```python
from build123d import *

# Parameters (mm, degrees)
F0_R        = 3
F1_DEPTH    = 3
F2_R        = 10
F3_R        = 5
F4_R        = 1
F5_T1_DEPTH = 3
F6_R        = 20
F7_R        = 1
F8_R        = 3
F9_R        = 8


# Not quite as in the source:
# - a fillet or chamfer that OpenCascade refuses, or shapes differently, is made with other operations: its cross-section is extruded or revolved along the edge and cut away or added
# - a feature names something its author has since deleted; it is built from what else it names


with BuildPart() as f1:
    # F0 (on Front) → F1 (new body)
    with BuildSketch(Plane.XZ):
        Polygon((-2, -2), (1.3333333333, 0), (0, 0), (0, 7), (-10, 2.5), (-10, -2), align=None)
        Polygon((14.2307692308, 0), (32, 0), (40, 0), (40, 7), (0, 7), (0, 0), (1.3333333333, 0), (8, 4), (13, 4), align=None)
        Polygon((15, -5), (32, 0), (14.2307692308, 0), (15, -2.5), (11.75, -3.5), align=None)
        with BuildLine():
            Line((40, 7), (40, 0))
            ThreePointArc((40, 0), (61.4283268073, 3.5), (40, 7))
        make_face()
        with Locations((57.4283268073, 3.5)):
            Circle(F0_R, mode=Mode.SUBTRACT)
    extrude(amount=F1_DEPTH)

    # F2
    f2_edges = [f1.edges().sort_by_distance(p)[0] for p in [
        (32, -1.5, 0),
    ]]
    fillet(f2_edges, radius=F2_R)

    # F3
    f3_edges = [f1.edges().sort_by_distance(p)[0] for p in [
        (13, -1.5, 4),
        (-2, -1.5, -2),
    ]]
    fillet(f3_edges, radius=F3_R)

    # F4
    f4_edges = [f1.edges().sort_by_distance(p)[0] for p in [
        (15, -1.5, -2.5),
    ]]
    fillet(f4_edges, radius=F4_R)

    # F5: fillet of radius 5 on 1 edges, made by hand

    # F5_s2 → F5_t1 (join)
    with BuildSketch(Plane.XZ):
        with BuildLine():
            ThreePointArc((9.3849198247, 4), (8.0502519153, 3.8185746411), (6.8124410476, 3.2874646286))
            Line((6.8124410476, 3.2874646286), (8, 4))
            Line((8, 4), (9.3849198247, 4))
        make_face()
    extrude(amount=F5_T1_DEPTH)

    # F6
    f6_edges = [f1.edges().sort_by_distance(p)[0] for p in [
        (0, -1.5, 7),
    ]]
    fillet(f6_edges, radius=F6_R)

    # F7
    f7_edges = [f1.edges().sort_by_distance(p)[0] for p in [
        (-10, -1.5, 2.5),
        (-10, -1.5, -2),
    ]]
    fillet(f7_edges, radius=F7_R)

    # F8
    f8_edges = [f1.edges().sort_by_distance(p)[0] for p in [
        (15, -1.5, -5),
    ]]
    fillet(f8_edges, radius=F8_R)

    # F9
    f9_edges = [f1.edges().sort_by_distance(p)[0] for p in [
        (40, -1.5, 7),
        (40, -1.5, 0),
    ]]
    fillet(f9_edges, radius=F9_R)


solid = f1.part
```
For this review, take the finished solid that the model builds, in its own axes (mm). A direction names the side the tool comes from. Round coordinates to 2 decimals unless told otherwise and drop trailing zeros. Write each loop counter-clockwise with the first axis right and the second up, starting at its lowest first coordinate (ties: lowest second). Pieces come first, ordered by that corner, then holes. Notation, with made-up numbers: (3.5, -3) -> (21.5, -3) arc R7 ccw to (21.5, 1) -> close; hole circle Ø11 at (19.25, 53.25). An arc over 180 degrees is marked (long way). One line per question, with ' | ' between items. Start each with the question number.
(1) Add section A-A, the plane y = -2.3. Write out the cut boundary in (x, z), plus the area to 3 significant figures.
(2) Add section D-D, the plane x = 0.5. Write out the cut boundary in (y, z), plus the area to 3 significant figures.
(3) Add section B-B, the plane x = 57. Write out the cut boundary in (y, z), plus the area to 3 significant figures.
(4) For line 1 along Z through (x, y) = (33, -2.35); line 2 along Z through (x, y) = (13, -1.1); line 3 along Z through (x, y) = (56.5, -2.5), list the stretches that pass through material, from the lowest coordinate up. Write a range as from..to.
(5) Mouldability with a two-part tool opening along Z and no side actions: class faces 6 (the face through (12.848, -1.479, -4.007)), 7 (the face through (12.329, -1.521, 2.984)), 8 (the face through (38.904, -1.521, 7.856)) as released by +Z, released by -Z, zero draft, split by the parting line, or undercut.
(6) Add section C-C, the plane z = 11.25. Write out the cut boundary in (x, y).
(7) Insertion check: P1, Ø1.5, axis at x = 34, y = -1, coming from the -Z side; P2, Ø1.5, axis at x = 23, y = -2, coming from the +Z side; P3, Ø1.5, axis at x = 52, y = -2.5, coming from the +Z side. Each pin has a flat end and moves straight along its axis. Give the tip position at first contact, or say it passes through.
(8) Tool access review of faces 1 (the face through (32.03, -1.52, -0.1)), 2 (the face through (-6, -1, -2)), 3 (the face through (20, -1, 7)), 4 (the face through (14.639, -1.521, -2.296)), 5 (the face through (12.913, -1.479, -3.142)): name each direction out of +Z, -Z, +X, -X, +Y, -Y from which nothing blocks a thin tool from reaching the whole face with its end or side.
Answer list:
1) outline: (-10, -1) arc R1 ccw to (-9, -2) -> (-3.38, -2) arc R5 ccw to (-0.81, -1.29) -> (6.81, 3.29) arc R5 cw to (9.35, 4) arc R5 cw to (14.09, 0.47) -> (14.71, -1.54) arc R1 cw to (14.04, -2.79) -> (11.75, -3.5) -> (13.98, -4.53) arc R3 ccw to (16.08, -4.68) -> (30.62, -0.41) arc R10 cw to (33.44, 0) -> (35.3, 0) arc R8 cw to (41.67, -3.16) arc R11 ccw (long way) to (41.67, 10.16) arc R8 cw to (35.3, 7) -> (4.29, 7) arc R20 ccw to (-3.91, 5.24) -> (-9.41, 2.77) arc R1 ccw to (-10, 1.85) -> close; hole circle Ø6 at (57.43, 3.5) | area: 715 mm²
2) outline: (-3, -0.5) -> (0, -0.5) -> (0, 6.64) -> (-3, 6.64) -> close | area: 21.4 mm²
3) outline: (-3, -5.32) -> (0, -5.32) -> (0, 0.53) -> (-3, 0.53) -> close; (-3, 6.47) -> (0, 6.47) -> (0, 12.32) -> (-3, 12.32) -> close | area: 35.1 mm²
4) line 1: -0.01..7 | line 2: -4.08..-3.12, 2.37..7 | line 3: -5.67..0.65, 6.35..12.67
5) face 6: released by -Z | face 7: undercut | face 8: released by +Z
6) outline: (42.62, -3) -> (58.23, -3) -> (58.23, 0) -> (42.62, 0) -> close
7) P1: z = 0 | P2: z = 7 | P3: z = 14.47
8) face 1: -Z, +Y, -Y | face 2: -Z, -X, +Y, -Y | face 3: +Z, -X, +Y, -Y | face 4: +Y, -Y | face 5: -X, +Y, -Y
